Check sheet for the modelled part. Datum: model origin and axes. Units: mm. A direction names the side the tool comes from. Round coordinates to 2 decimals unless told otherwise and drop trailing zeros. Order: outer loops, then holes, each group sorted by start corner. A loop starts at its lowest first (then second) coordinate and runs counter-clockwise, first axis right, second up.
from build123d import *

# Parameters (mm, degrees)
F0_W      = 250
F0_H      = 250
F1_DEPTH  = 1000
F2_T      = -50
F3_W      = 1150
F3_H      = 120
F4_DEPTH  = 1100
F5_W      = 900
F5_H      = 200
F6_DEPTH  = 5000
F7_W      = 900
F7_H      = 200
F8_DEPTH  = 300
F9_W      = 900
F9_H      = 200
F10_DEPTH = 300
F11_W     = 900
F11_H     = 200
F12_DEPTH = 300
F13_W     = 900
F13_H     = 200
F14_DEPTH = 300
F15_W     = 900
F15_H     = 200
F16_DEPTH = 300
F17_W     = 150
F17_H     = 200
F17_W_2   = 558.2895040512
F17_H_2   = 530
F17_W_3   = 147.1817493439
F17_H_3   = 30
F18_DEPTH = 5000


with BuildPart() as f1:
    # F0 (on Front) → F1 (new body)
    with BuildSketch(Plane.XZ):
        Polygon((0, 250), (0, 0), (1250, 0), (1250, 250), (1050, 250), align=None)
        Polygon((0, 500), (0, 250), (1050, 250), (1050, 500), (850, 500), align=None)
        Polygon((0, 750), (0, 500), (850, 500), (850, 750), (650, 750), align=None)
        Polygon((0, 1000), (0, 750), (650, 750), (650, 1000), (450, 1000), align=None)
        Polygon((0, 1250), (0, 1000), (450, 1000), (450, 1250), (250, 1250), align=None)
        with Locations((125, 1375)):
            Rectangle(F0_W, F0_H)
    extrude(amount=F1_DEPTH)

    # F2
    f2_openings = [f1.faces().sort_by_distance(p)[0] for p in [
        (0, -500, 750),
    ]]
    offset(amount=F2_T, openings=f2_openings, kind=Kind.INTERSECTION)

    # F3 (on face) → F4 (cut)
    with BuildSketch(Plane.XZ.offset(1000)):
        with Locations((625, 60)):
            Rectangle(F3_W, F3_H)
    extrude(amount=-F4_DEPTH, mode=Mode.SUBTRACT)

    # F5 (on face) → F6 (cut)
    with BuildSketch(Plane.YZ.offset(1250)):
        with Locations((-500, 100)):
            Rectangle(F5_W, F5_H)
    extrude(amount=-F6_DEPTH, mode=Mode.SUBTRACT)

    # F7 (on face) → F8 (cut)
    with BuildSketch(Plane.YZ.offset(1050)):
        with Locations((-500, 350)):
            Rectangle(F7_W, F7_H)
    extrude(amount=-F8_DEPTH, mode=Mode.SUBTRACT)

    # F9 (on face) → F10 (cut)
    with BuildSketch(Plane.YZ.offset(850)):
        with Locations((-500, 600)):
            Rectangle(F9_W, F9_H)
    extrude(amount=-F10_DEPTH, mode=Mode.SUBTRACT)

    # F11 (on face) → F12 (cut)
    with BuildSketch(Plane.YZ.offset(650)):
        with Locations((-500, 850)):
            Rectangle(F11_W, F11_H)
    extrude(amount=-F12_DEPTH, mode=Mode.SUBTRACT)

    # F13 (on face) → F14 (cut)
    with BuildSketch(Plane.YZ.offset(450)):
        with Locations((-500, 1100)):
            Rectangle(F13_W, F13_H)
    extrude(amount=-F14_DEPTH, mode=Mode.SUBTRACT)

    # F15 (on face) → F16 (cut)
    with BuildSketch(Plane.YZ.offset(250)):
        with Locations((-500, 1350)):
            Rectangle(F15_W, F15_H)
    extrude(amount=-F16_DEPTH, mode=Mode.SUBTRACT)

    # F17 (on face) → F18 (cut)
    with BuildSketch(Plane(origin=(0, 0, 0), x_dir=(-1, 0, 0), z_dir=(0, 1, 0))):
        with Locations((-525, 850)):
            Rectangle(F17_W, F17_H)
        Polygon((-200, 750), (-50, 750), (-50, 1450), (-200, 1450), (-200, 1200), align=None)
        Polygon((-250, 750), (-250, 1200), (-400, 1200), (-400, 950), (-400, 750), align=None)
        with Locations((-329.1447520256, 435)):
            Rectangle(F17_W_2, F17_H_2)
        Polygon((-658.2895040512, 700), (-800, 700), (-800, 450), (-800, 170), (-658.2895040512, 170), align=None)
        Polygon((-850, 170), (-850, 450), (-1000, 450), (-1000, 200), (-1000, 170), align=None)
        with Locations((-1126.4091253281, 185)):
            Rectangle(F17_W_3, F17_H_3)
    extrude(amount=-F18_DEPTH, mode=Mode.SUBTRACT)


solid = f1.part
1) Set-up check for faces 1 (the face through (25, -25, 0)), 2 (the face through (658.29, -975, 431)), 3 (the face through (50, -25, 59)): record each of +Z, -Z, +X, -X, +Y, -Y from which the full face is reachable in a straight line by a thin tool's end or side.
2) Sectioned sample at A-A on y = -539.5. Record the cut outline in (x, z).
3) Scan lines: line 1 (X direction, y = -959, z = 839); line 2 (Z direction, x = 804, y = -889); line 3 (Z direction, x = 610.5, y = -81). Record each from-to range of solid material in increasing order.
4) Sectioned sample at B-B on x = 1026.5. Record the cut outline in (y, z), and give its area (3 significant figures).
5) Draft check along X on faces 4 (the face through (526, -25, 750)), 5 (the face through (628, -50, 507)), 6 (the face through (50, -975, 59)), 7 (the face through (450, -609, 1208)). Enter one of: pulls with the +X half, pulls with the -X half, needs draft (parallel to the pull), parting line crosses it, or undercut.
6) Sectioned sample at C-C on x = 877. Record the cut outline in (y, z), and give its area (3 significant figures).
7) Sectioned sample at D-D on x = 153.5. Record the cut outline in (y, z), and give its area (3 significant figures).
8) Gauge pin test, flat ends, axial feed: pin 1 (6 mm diameter, centred on y = -200, z = 701.5, fed in from +X); pin 2 (3 mm diameter, centred on x = 419, y = -830.5, fed in from +Z); pin 3 (6 mm diameter, centred on x = 537, y = -762.5, fed in from -Z); pin 4 (2 mm diameter, centred on x = 451.5, z = 752.5, fed in from +Y). Record the tip position at first contact, or that the pin passes through.
Values found:
1. face 1: -Z, +X, -X, +Y, -Y
1. face 2: +Y, -Y
1. face 3: -Z, +Y, -Y
2. outline: (0, 1450) - (250, 1450) - (250, 1500) - (0, 1500) - close; (200, 1200) - (450, 1200) - (450, 1250) - (200, 1250) - close; (400, 950) - (650, 950) - (650, 1000) - (400, 1000) - close; (600, 700) - (850, 700) - (850, 750) - (600, 750) - close; (800, 450) - (1050, 450) - (1050, 500) - (800, 500) - close; (1000, 200) - (1250, 200) - (1250, 250) - (1000, 250) - close
3. line 1: x = 0 to 50, 200 to 250, 400 to 450, 600 to 650
3. line 2: z = 450 to 500, 700 to 750
3. line 3: z = 700 to 750, 950 to 1000
4. outline: (-1000, 120) - (-950, 120) - (-950, 200) - (-50, 200) - (-50, 120) - (0, 120) - (0, 500) - (-1000, 500) - close; hole (-950, 250) - (-50, 250) - (-50, 450) - (-950, 450) - close
4. area: 128,000 mm2
5. face 4: undercut
5. face 5: needs draft
5. face 6: undercut
5. face 7: pulls with the +X half
6. outline: (-1000, 120) - (-950, 120) - (-950, 170) - (-1000, 170) - close; (-1000, 450) - (0, 450) - (0, 500) - (-1000, 500) - close; (-50, 120) - (0, 120) - (0, 170) - (-50, 170) - close
6. area: 55,000 mm2
7. outline: (-1000, 120) - (-950, 120) - (-950, 170) - (-1000, 170) - close; (-1000, 700) - (-950, 700) - (-950, 750) - (-1000, 750) - close; (-1000, 1450) - (0, 1450) - (0, 1500) - (-1000, 1500) - close; (-50, 120) - (0, 120) - (0, 170) - (-50, 170) - close; (-50, 700) - (0, 700) - (0, 750) - (-50, 750) - close
7. area: 60,000 mm2
8. pin 1: stops at x = 850
8. pin 2: stops at z = 1250
8. pin 3: stops at z = 950
8. pin 4: passes through
